Could you check a few things on this model? Use its own coordinates, in mm. Face numbers are marked on the shaded views. Coordinates: 2 decimals unless noted, no trailing zeros. Loops run counter-clockwise (first coordinate to the right, second up) from the corner with the lowest first, then second, coordinate; pieces in that order, holes last. Notation, with made-up numbers: (5, -20.75) -> (21, -20.75) arc R3 cw to (21, -15.75) -> close; hole circle Ø4 at (46.25, 45). An arc over 180 degrees is marked (long way). One line per question, with ' | ' between items.
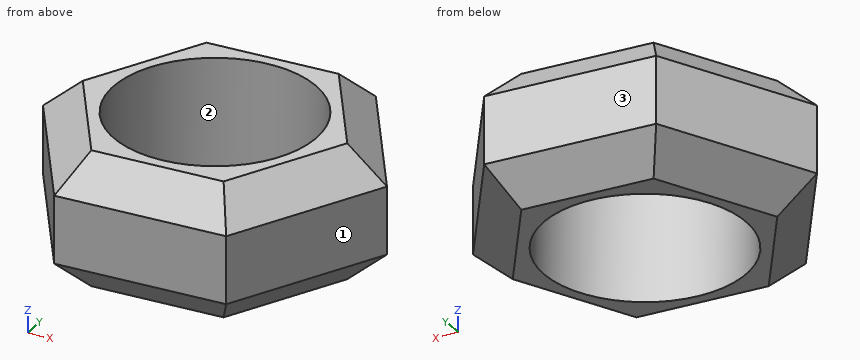
from build123d import *

# Parameters (mm, degrees)
F0_R     = 15
F1_DEPTH = 20
F2_R     = 15
F3_DEPTH = 33.7
F4_SIZE  = 5


with BuildPart() as f1:
    # F0 (on Top) → F1 (new body)
    with BuildSketch(Plane.XY):
        Circle(F0_R)
        Polygon((-11.400712, -22.249129), (13.567955, -20.997871), (24.968667, 1.251258), (11.400712, 22.249129), (-13.567955, 20.997871), (-24.968667, -1.251258), align=None)
        Circle(F0_R, mode=Mode.SUBTRACT)
    extrude(amount=F1_DEPTH)

    # F2 (on face) → F3 (cut)
    with BuildSketch(Plane(origin=(0, 0, 0), x_dir=(1, 0, 0), z_dir=(0, 0, -1))):
        Circle(F2_R)
    extrude(amount=-F3_DEPTH, mode=Mode.SUBTRACT)

    # F4
    f4_edges = [f1.edges().sort_by_distance(p)[0] for p in [
        (1.083621, -21.6235, 20),
        (1.083621, -21.6235, 0),
        (-18.18469, -11.750194, 0),
        (-18.18469, -11.750194, 20),
        (-19.268311, 9.873307, 0),
        (-19.268311, 9.873307, 20),
        (-1.083621, 21.6235, 20),
        (-1.083621, 21.6235, 0),
        (18.18469, 11.750194, 0),
        (18.18469, 11.750194, 20),
        (19.268311, -9.873307, 20),
        (19.268311, -9.873307, 0),
    ]]
    chamfer(f4_edges, length=F4_SIZE)


solid = f1.part
1) I need wall thicknesses on line 1 along Y through (x, z) = (-9, 16.75); line 2 along X through (y, z) = (5.5, 6.5); line 3 along Y through (x, z) = (0, 11.5). Which ranges of each line are inside material? Lowest first, please. Write a range as from..to.
Data:
line 1: -20.38..-12, 12..19.47 | line 2: -21.51..-13.96, 13.96..22.22 | line 3: -21.68..-15, 15..21.68
2) If we section it at D-D on x = 17: Please give me the cut outline in (y, z), and give its area (3 significant figures).
Data:
outline: (-14.3, 5) -> (-3.34, 0) -> (4.37, 0) -> (13.58, 5) -> (13.58, 15) -> (4.37, 20) -> (-3.34, 20) -> (-14.3, 15) -> close | area: 457 mm²
3) If we section it at A-A on y = 4: Please give me the cut outline in (x, z), and give its area (3 significant figures).
Data:
outline: (-22.28, 5) -> (-16.66, 0) -> (-14.46, 0) -> (-14.46, 20) -> (-16.66, 20) -> (-22.28, 15) -> close; (14.46, 0) -> (17.24, 0) -> (23.19, 5) -> (23.19, 15) -> (17.24, 20) -> (14.46, 20) -> close | area: 273 mm²
4) I'm going to push flat-ended pins straight in: pin 1 Ø12 at (x, z) = (-5, 16) entering from +Y; pin 2 Ø8 at (x, z) = (15, 16) entering from -Y; pin 3 Ø5 at (x, z) = (5, 11.5) entering from -Y. Where does each tip first touch, or does it pass through?
Data:
pin 1: y = 21.72 | pin 2: y = -21.12 | pin 3: y = -21.55
5) If we section it at C-C on x = 0: Please give me the cut outline in (y, z).
Data:
outline: (-21.68, 5) -> (-16.67, 0) -> (-15, 0) -> (-15, 20) -> (-16.67, 20) -> (-21.68, 15) -> close; (15, 0) -> (16.67, 0) -> (21.68, 5) -> (21.68, 15) -> (16.67, 20) -> (15, 20) -> close
6) We'd pull the mould along X, two halves only. Please class the marked faces 1, 2 and 3: pulls with the +X half, pulls with the -X half, needs draft (parallel to the pull), parting line crosses it, or undercut.
Data:
face 1: pulls with the +X half | face 2: undercut | face 3: pulls with the -X half
7) If we section it at B-B on z = 10.5: Please give me the cut outline in (x, y), and give its area (3 significant figures).
Data:
outline: (-24.97, -1.25) -> (-11.4, -22.25) -> (13.57, -21) -> (24.97, 1.25) -> (11.4, 22.25) -> (-13.57, 21) -> close; hole circle Ø30 at (0, 0) | area: 917 mm²
